Read the model definition and answer for the solid it produces. Units are mm, in the model's axes. Face numbers are marked on the shaded views. A direction names the side the tool comes from. Round coordinates to 2 decimals unless told otherwise and drop trailing zeros. Order: outer loops, then holes, each group sorted by start corner. A loop starts at its lowest first (then second) coordinate and runs counter-clockwise, first axis right, second up. Notation, with made-up numbers: (26.5, 73) - (39.5, 73) arc R10 ccw to (39.5, 80) - close; hole circle Ø10 at (-27.75, -37). An arc over 180 degrees is marked (long way). Put each result on its own line as item: value. Start each with the question number.
Q1. Each of these flat-tipped pins is pushed along its axis until it touches: pin 1 Ø2.5 at (x, y) = (-97.5, 22.65) entering from +Z; pin 2 Ø3 at (x, y) = (-24, 27.5) entering from +Z; pin 3 Ø2 at (y, z) = (15.5, -39) entering from +X; pin 4 Ø4 at (x, y) = (93.5, 42.65) entering from -Z. Where does it stop, or does it pass through?
Q2. Section D-D on y = 28 is taken. Give the vertices of the cut face in (x, z), then the cut area to 3 significant figures.
Q3. Section B-B on z = -15 is taken. Give the vertices of the cut face in (x, y).
Q4. Section A-A on y = 39 is taken. Give the vertices of the cut face in (x, z), then the cut area to 3 significant figures.
Q5. Find the intervals of material crossed by line 1 along Y through (x, z) = (-97.5, -54.4); line 2 along Y through (x, z) = (93.5, -54.35); line 3 along X through (y, z) = (42, -54), in increasing order. Write a range as from..to.
Q6. Section C-C on x = -28 is taken. Give the vertices of the cut face in (y, z).
Q7. Which of the six approach directions +Z, -Z, +X, -X, +Y, -Y give full straight-line access (tool end or side, diameter ignored) to the marked faces 1, 2 and 3?
from build123d import *

# Parameters (mm, degrees)
SKETCH1_W                    = 199
SKETCH1_H                    = 110
BASE_FLANGE1_DEPTH           = 1.35
EDGE_FLANGE1_STRIP_W         = 6.4
EDGE_FLANGE1_STRIP_H         = 1.35
EDGE_FLANGE1_STRIP_CUT_DEPTH = 199
EDGE_FLANGE1_DEPTH           = 199
EDGE_FLANGE2_START           = -55
EDGE_FLANGE2_DEPTH           = 97.675
EDGE_FLANGE2_2_DEPTH         = 1.85
EDGE_FLANGE2_START_2         = 42
EDGE_FLANGE2_3_DEPTH         = 0.675
EDGE_FLANGE2_START_3         = -53.15
EDGE_FLANGE2_4_DEPTH         = 95.15
JOG1_START                   = -53.15
JOG1_DEPTH                   = 95.15
JOG1_2_DEPTH                 = 95.15
SKETCH13_W                   = 2
SKETCH13_H                   = 10
CUT_EXTRUDE1_DEPTH           = 10
SKETCH15_R                   = 1.5
CUT_EXTRUDE2_DEPTH           = 10
SKETCH31_W                   = 9
SKETCH31_H                   = 28.176598128
BOSS_EXTRUDE2_DEPTH          = 1.35
CUT_EXTRUDE3_DEPTH           = 124.661119597


# Read off the part's stored shape, not the designer's step: Edge-Flange2, Jog1
# Sheet-metal steps are written as plain solids
with BuildPart() as part:
    # Sketch1 → Base-Flange1 (new body)
    with BuildSketch(Plane(origin=(0, 0, 0), x_dir=(1, 0, 0), z_dir=(0, 1, 0))):
        Rectangle(SKETCH1_W, SKETCH1_H)
    extrude(amount=-BASE_FLANGE1_DEPTH)

    # Edge-Flange1 strip (across the edge) → Edge-Flange1 strip cut (cut)
    with BuildSketch(Plane(origin=(99.5, 0, -55), x_dir=(0, 0, 1), z_dir=(-1, 0, 0))):
        with Locations((-1.35, -0.675)):
            Rectangle(EDGE_FLANGE1_STRIP_W, EDGE_FLANGE1_STRIP_H)
    extrude(amount=EDGE_FLANGE1_STRIP_CUT_DEPTH, mode=Mode.SUBTRACT)

    # Edge-Flange1 section (across the edge) → Edge-Flange1 (add)
    with BuildSketch(Plane(origin=(99.5, 0, -55), x_dir=(0, 0, 1), z_dir=(-1, 0, 0))):
        with BuildLine():
            Line((0, 0.5), (0, 48.65))
            Line((0, 48.65), (1.35, 48.65))
            Line((1.35, 48.65), (1.35, 0.5))
            ThreePointArc((1.35, 0.5), (1.496446609, 0.146446609), (1.85, 0))
            Line((1.85, 0), (1.85, -1.35))
            ThreePointArc((1.85, -1.35), (0.541852455, -0.808147545), (0, 0.5))
        make_face()
    extrude(amount=EDGE_FLANGE1_DEPTH)

    # Edge-Flange2 outline → Edge-Flange2 (cut)
    with BuildSketch(Plane.XY.offset(EDGE_FLANGE2_START)):
        with BuildLine():
            Line((-97.65, 0), (-97.65, 0.5))
            Line((-97.65, 0.5), (-98.15, 0.5))
            ThreePointArc((-98.15, 0.5), (-98.003553391, 0.146446609), (-97.65, 0))
        make_face()
        with BuildLine():
            Line((-99.5, 0.5), (-99.5, -1.35))
            Line((-99.5, -1.35), (-97.65, -1.35))
            ThreePointArc((-97.65, -1.35), (-98.958147545, -0.808147545), (-99.5, 0.5))
        make_face()
    extrude(amount=EDGE_FLANGE2_DEPTH, mode=Mode.SUBTRACT)

    # Edge-Flange2 2 outline → Edge-Flange2 2 (cut)
    with BuildSketch(Plane.XY.offset(EDGE_FLANGE2_START)):
        with BuildLine():
            ThreePointArc((-97.65, 0), (-98.003553391, 0.146446609), (-98.15, 0.5))
            Line((-98.15, 0.5), (-99.5, 0.5))
            ThreePointArc((-99.5, 0.5), (-98.958147545, -0.808147545), (-97.65, -1.35))
            Line((-97.65, -1.35), (-97.65, 0))
        make_face()
    extrude(amount=EDGE_FLANGE2_2_DEPTH, mode=Mode.SUBTRACT)

    # Edge-Flange2 3 outline → Edge-Flange2 3 (cut)
    with BuildSketch(Plane.XY.offset(EDGE_FLANGE2_START_2)):
        with BuildLine():
            Line((-96.975, 0), (-99.431151313, 0))
            ThreePointArc((-99.431151313, 0), (-98.767474832, -0.97436427), (-97.65, -1.35))
            Line((-97.65, -1.35), (-96.975, -1.35))
            Line((-96.975, -1.35), (-96.975, 0))
        make_face()
    extrude(amount=EDGE_FLANGE2_3_DEPTH, mode=Mode.SUBTRACT)

    # Edge-Flange2 4 outline → Edge-Flange2 4 (add)
    with BuildSketch(Plane.XY.offset(EDGE_FLANGE2_START_3)):
        with BuildLine():
            ThreePointArc((-97.65, 0), (-98.003553391, 0.146446609), (-98.15, 0.5))
            Line((-98.15, 0.5), (-98.15, 44.65))
            Line((-98.15, 44.65), (-99.5, 44.65))
            Line((-99.5, 44.65), (-99.5, 0.5))
            ThreePointArc((-99.5, 0.5), (-99.482707004, 0.247641058), (-99.431151313, 0))
            Line((-99.431151313, 0), (-97.65, 0))
        make_face()
    extrude(amount=EDGE_FLANGE2_4_DEPTH)

    # Jog1 outline → Jog1 (cut)
    with BuildSketch(Plane.XY.offset(JOG1_START)):
        with BuildLine():
            Line((-99.5, 44.65), (-99.5, 7.65))
            ThreePointArc((-99.5, 7.65), (-99.359177135, 8.35796435), (-98.958147545, 8.958147545))
            Line((-98.958147545, 8.958147545), (-98.15, 9.76629509))
            Line((-98.15, 9.76629509), (-98.15, 44.65))
            Line((-98.15, 44.65), (-99.5, 44.65))
        make_face()
    extrude(amount=JOG1_DEPTH, mode=Mode.SUBTRACT)

    # Jog1 2 outline → Jog1 2 (add)
    with BuildSketch(Plane.XY.offset(JOG1_START)):
        with BuildLine():
            Line((-91.796446609, 16.119848481), (-98.15, 9.76629509))
            Line((-98.15, 9.76629509), (-98.15, 7.65))
            ThreePointArc((-98.15, 7.65), (-98.111939766, 7.841341716), (-98.003553391, 8.003553391))
            Line((-98.003553391, 8.003553391), (-90.841852455, 15.165254326))
            ThreePointArc((-90.841852455, 15.165254326), (-90.440822865, 15.765437522), (-90.3, 16.473401872))
            Line((-90.3, 16.473401872), (-90.3, 44.65))
            Line((-90.3, 44.65), (-91.65, 44.65))
            Line((-91.65, 44.65), (-91.65, 16.473401872))
            ThreePointArc((-91.65, 16.473401872), (-91.688060234, 16.282060156), (-91.796446609, 16.119848481))
        make_face()
    extrude(amount=JOG1_2_DEPTH)

    # Sketch13 → Cut-Extrude1 (cut)
    with BuildSketch(Plane.ZY.offset(99.5)):
        with Locations((-52.15, 39.65)):
            Rectangle(SKETCH13_W, SKETCH13_H)
    extrude(amount=-CUT_EXTRUDE1_DEPTH, mode=Mode.SUBTRACT)

    # Sketch15 → Cut-Extrude2 (cut)
    with BuildSketch(Plane.XY.offset(-53.65)):
        with Locations((-97.5, 42.65)):
            Circle(SKETCH15_R)
        with Locations((-97.5, 22.65)):
            Circle(SKETCH15_R)
        with Locations((93.5, 42.65)):
            Circle(SKETCH15_R)
        with Locations((93.5, 32.65)):
            Circle(SKETCH15_R)
    extrude(amount=-CUT_EXTRUDE2_DEPTH, mode=Mode.SUBTRACT)

    # Sketch31 → Boss-Extrude2 (add)
    with BuildSketch(Plane.ZY.offset(91.65)):
        with Locations((46.5, 30.561700936)):
            Rectangle(SKETCH31_W, SKETCH31_H)
    extrude(amount=-BOSS_EXTRUDE2_DEPTH)

    # Sketch16 → Cut-Extrude3 (cut, through all)
    with BuildSketch(Plane(origin=(0, 0, 0), x_dir=(1, 0, 0), z_dir=(0, 1, 0))):
        with BuildLine():
            Line((-96.5, -47.5), (-99.5, -47.5))
            Line((-99.5, -47.5), (-99.5, -50.5))
            Line((-99.5, -50.5), (-96.5, -50.5))
            ThreePointArc((-96.5, -50.5), (-95, -49), (-96.5, -47.5))
        make_face()
    extrude(amount=-CUT_EXTRUDE3_DEPTH, mode=Mode.SUBTRACT)


solid = part.part
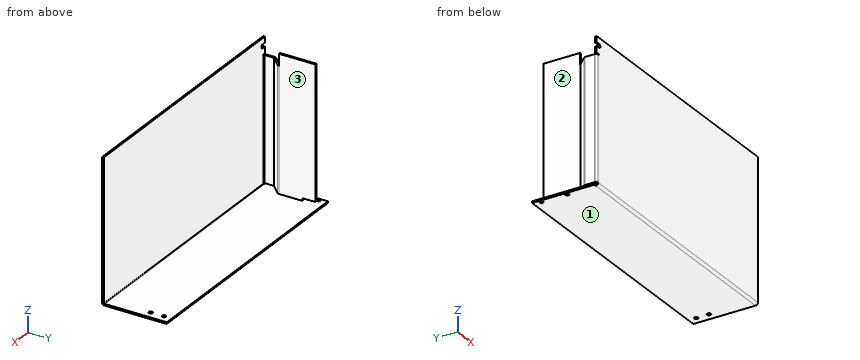
Findings:
1. pin 1: through
1. pin 2: z = -53.65
1. pin 3: x = -90.3
1. pin 4: z = -55
2. outline: (-99.5, -55) - (99.5, -55) - (99.5, -53.65) - (-99.5, -53.65) - close; (-91.65, -53.15) - (-90.3, -53.15) - (-90.3, 51) - (-91.65, 51) - close
2. area: 409 mm2
3. outline: (-99.5, 0.5) arc R1.85 ccw to (-97.65, -1.35) - (99.5, -1.35) - (99.5, 0) - (-97.65, 0) arc R0.5 cw to (-98.15, 0.5) - (-98.15, 7.65) arc R0.5 cw to (-98, 8) - (-90.84, 15.17) arc R1.85 ccw to (-90.3, 16.47) - (-90.3, 44.65) - (-91.65, 44.65) - (-91.65, 16.47) arc R0.5 cw to (-91.8, 16.12) - (-98.96, 8.96) arc R1.85 ccw to (-99.5, 7.65) - close
4. outline: (-99.5, -55) - (99.5, -55) - (99.5, -53.65) - (-99.5, -53.65) - close; (-91.65, -51.15) - (-90.3, -51.15) - (-90.3, 51) - (-91.65, 51) - close
4. area: 407 mm2
5. line 1: -0.86..21.15, 24.15..41.15, 44.15..48.65
5. line 2: -0.91..31.15, 34.15..41.15, 44.15..48.65
5. line 3: -99.5..-98.85, -96.15..92.15, 94.85..99.5
6. outline: (-1.35, -53.15) arc R1.85 ccw to (0.5, -55) - (48.65, -55) - (48.65, -53.65) - (0.5, -53.65) arc R0.5 cw to (0, -53.15) - (0, 55) - (-1.35, 55) - close
7. face 1: -Z, +X, -X, +Y, -Y
7. face 2: +Z, -X, +Y
7. face 3: +Z, +X, +Y
